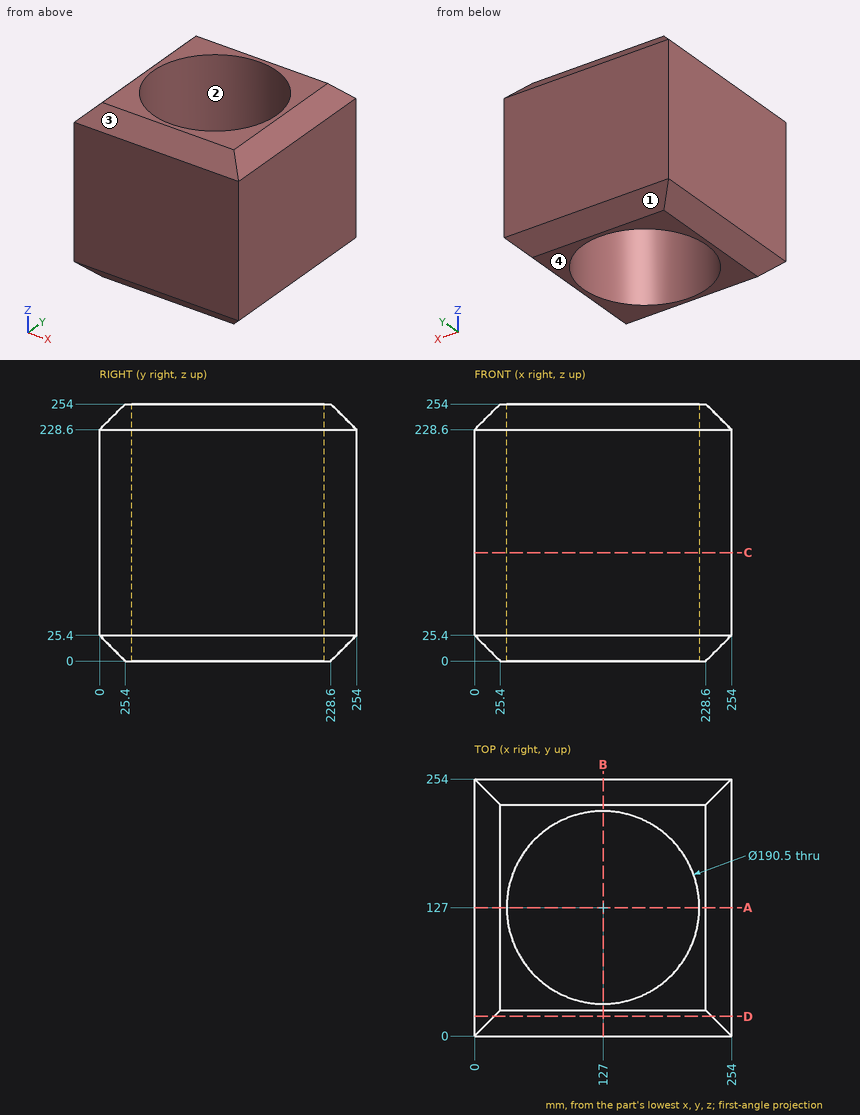
Geometry check sheet. Reference: drawing and pictorial views, mm from the part's lowest x, y, z. Round coordinates to 2 decimals unless told otherwise and drop trailing zeros. Loops run counter-clockwise (first coordinate to the right, second up) from the corner with the lowest first, then second, coordinate; pieces in that order, holes last. Notation, with made-up numbers: (76, 80) - (130, 80) arc R16 ccw to (130, 90) - close; hole circle Ø1 at (-26.75, 31.25). An arc over 180 degrees is marked (long way). Write item = value, one per line. Start each with the question number.
Q1. Section check C-C (z = 107). Record the boundary of the cut face in (x, y).
Q2. Section check A-A (y = 127). Record the boundary of the cut face in (x, z).
Q3. Release check for a two-part mould opening along Y. For the marked faces 1, 2, 3 and 4 record: pulls with the +Y half, pulls with the -Y half, needs draft (parallel to the pull), parting line crosses it, or undercut.
Q4. Thickness scan on L1, parallel to Y at x = 127, z = 130; L2, parallel to Y at x = 108.5, z = 52; L3, parallel to X at y = 38.5, z = 85.5. Record the ranges inside material, lowest first.
Q5. Section check D-D (y = 19.5). Record the boundary of the cut face in (x, z).
Derived:
q1.outline = (0, 0) - (254, 0) - (254, 254) - (0, 254) - close; hole circle Ø190.5 at (127, 127)
q2.outline = (0, 25.4) - (25.4, 0) - (31.75, 0) - (31.75, 254) - (25.4, 254) - (0, 228.6) - close; (222.25, 0) - (228.6, 0) - (254, 25.4) - (254, 228.6) - (228.6, 254) - (222.25, 254) - close
q3.face_1 = pulls with the +Y half
q3.face_2 = undercut
q3.face_3 = pulls with the -Y half
q3.face_4 = needs draft
q4.L1 = 0 to 31.75, 222.25 to 254
q4.L2 = 0 to 33.56, 220.44 to 254
q4.L3 = 0 to 91.78, 162.22 to 254
q5.outline = (0, 25.4) - (19.5, 5.9) - (234.5, 5.9) - (254, 25.4) - (254, 228.6) - (234.5, 248.1) - (19.5, 248.1) - (0, 228.6) - close
